Here's how the part is built. I have some questions about the finished solid (model axes, mm). A direction names the side the tool comes from. Round coordinates to 2 decimals unless told otherwise and drop trailing zeros. Loops run counter-clockwise (first coordinate to the right, second up) from the corner with the lowest first, then second, coordinate; pieces in that order, holes last. Notation, with made-up numbers: M 23,34.5 L 35,34.5 A15 cw 35,49.5 Z; hole C 27,-14 d10. An arc over 180 degrees is marked long. Use a Markdown table: item, result.
```python
from build123d import *

# Parameters (mm, degrees)
SKETCH1_W                                      = 45
SKETCH1_H                                      = 35
BOSS_EXTRUDE1_DEPTH                            = 3
CSK_FOR_M3_FLAT_HEAD_MACHINE_SCREW2_AT_2_COUNT = 2
CSK_FOR_M3_FLAT_HEAD_MACHINE_SCREW2_AT_2_PITCH = 20
CSK_FOR_M3_FLAT_HEAD_MACHINE_SCREW2_AT_3_COUNT = 2
CSK_FOR_M3_FLAT_HEAD_MACHINE_SCREW2_AT_3_PITCH = 28.284271247
CSK_FOR_M3_FLAT_HEAD_MACHINE_SCREW2_AT_4_COUNT = 2
CSK_FOR_M3_FLAT_HEAD_MACHINE_SCREW2_AT_4_PITCH = 20
SKETCH7_W                                      = 10
SKETCH7_H                                      = 4
BOSS_EXTRUDE2_DEPTH                            = 50
FILLET1_R                                      = 2
SKETCH12_W                                     = 10
SKETCH12_H                                     = 10
BOSS_EXTRUDE3_DEPTH                            = 15


with BuildPart() as part:
    # Sketch1 → Boss-Extrude1 (new body)
    with BuildSketch(Plane(origin=(0, 0, 0), x_dir=(1, 0, 0), z_dir=(0, 1, 0))):
        Rectangle(SKETCH1_W, SKETCH1_H)
    extrude(amount=BOSS_EXTRUDE1_DEPTH)

    # Sketch5 → CSK for M3 Flat Head Machine Screw2 (revolve, cut)
    with BuildSketch(Plane(origin=(10, 3, -10), x_dir=(0, 0, 1), z_dir=(1, 0, 0))):
        Polygon((0, 0), (0, 3), (1.7, 3), (1.7, 1.45), (3.15, 0), align=None)
    csk_for_m3_flat_head_machine_screw2 = revolve(axis=Axis((10, 9.35, -10), (0, -1, 0)), mode=Mode.SUBTRACT)

    # CSK for M3 Flat Head Machine Screw2 at 2: CSK for M3 Flat Head Machine Screw2 ×2
    with Locations(*[(-i * CSK_FOR_M3_FLAT_HEAD_MACHINE_SCREW2_AT_2_PITCH, 0, 0) for i in range(1, CSK_FOR_M3_FLAT_HEAD_MACHINE_SCREW2_AT_2_COUNT)]):
        add(csk_for_m3_flat_head_machine_screw2, mode=Mode.SUBTRACT)

    # CSK for M3 Flat Head Machine Screw2 at 3: CSK for M3 Flat Head Machine Screw2 ×2
    with Locations(*[Vector(-0.707106781, 0, 0.707106781) * (i * CSK_FOR_M3_FLAT_HEAD_MACHINE_SCREW2_AT_3_PITCH) for i in range(1, CSK_FOR_M3_FLAT_HEAD_MACHINE_SCREW2_AT_3_COUNT)]):
        add(csk_for_m3_flat_head_machine_screw2, mode=Mode.SUBTRACT)

    # CSK for M3 Flat Head Machine Screw2 at 4: CSK for M3 Flat Head Machine Screw2 ×2
    with Locations(*[(0, 0, i * CSK_FOR_M3_FLAT_HEAD_MACHINE_SCREW2_AT_4_PITCH) for i in range(1, CSK_FOR_M3_FLAT_HEAD_MACHINE_SCREW2_AT_4_COUNT)]):
        add(csk_for_m3_flat_head_machine_screw2, mode=Mode.SUBTRACT)

    # Sketch7 → Boss-Extrude2 (add, along a direction that is not the sketch's normal)
    with BuildSketch(Plane(origin=(0, 3, 0), x_dir=(1, 0, 0), z_dir=(0, 1, 0))):
        Rectangle(SKETCH7_W, SKETCH7_H)
    extrude(amount=BOSS_EXTRUDE2_DEPTH, dir=(0, 0.866025404, -0.5))

    # Fillet1
    fillet1_edges = [part.edges().sort_by_distance(p)[0] for p in [
        (22.5, 3, 0),
        (0, 3, -17.5),
        (-22.5, 3, 0),
        (0, 3, 17.5),
        (-22.5, 1.5, -17.5),
        (22.5, 1.5, -17.5),
        (22.5, 1.5, 17.5),
        (-22.5, 1.5, 17.5),
    ]]
    fillet(fillet1_edges, radius=FILLET1_R)

    # Sketch12 → Boss-Extrude3 (add)
    with BuildSketch(Plane(origin=(0, 3, 0), x_dir=(1, 0, 0), z_dir=(0, 1, 0))):
        with Locations((0, 3)):
            Rectangle(SKETCH12_W, SKETCH12_H)
    extrude(amount=BOSS_EXTRUDE3_DEPTH)


solid = part.part
```
Q1. We'd pull the mould along Z, two halves only. Please class faces 1 (the cylindrical face through (21.9, 0.51, -16.93)), 2 (the cylindrical face through (11.5, 0.8, -9.2)), 3 (the cylindrical face through (21.9, 2.43, -0.22)): pulls with the +Z half, pulls with the -Z half, needs draft (parallel to the pull), parting line crosses it, or undercut.
Return value:
| item | result |
|---|---|
| face 1 | pulls with the -Z half |
| face 2 | undercut |
| face 3 | needs draft |
Q2. Imagine slicing it at D-D, the plane x = -1. Please give me the cut outline in (y, z).
Return value:
| item | result |
|---|---|
| outline | M 0,-17.5 L 1,-17.5 A2 ccw 3,-15.5 L 3,-8 L 13.39,-8 L 46.3,-27 L 46.3,-23 L 18,-6.66 L 18,2 L 3,2 L 3,15.5 A2 ccw 1,17.5 L 0,17.5 Z |
Q3. For faces 4 (the cylindrical face through (21.9, 0.51, 16.93)), 5 (the flat face through (0, 10, 2)), 6 (the flat face through (-5, 21, -9)), 7 (the cylindrical face through (0.29, 2.4, -16.93)), which set-ups out of +Z, -Z, +X, -X, +Y, -Y let a thin tool reach every point of the face, with its end or its side?
Return value:
| item | result |
|---|---|
| face 4 | +Z, +X, +Y, -Y |
| face 5 | +Z, +X, -X, +Y |
| face 6 | +Z, -Z, -X, +Y |
| face 7 | -Z, +X, -X |
Q4. Imagine slicing it at A-A, the plane z = 10. Please give me the cut outline in (x, y).
Return value:
| item | result |
|---|---|
| outline | M -22.5,0 L -11.7,0 L -11.7,1.55 L -13.15,3 L -20.5,3 A2 ccw -22.5,1 Z; M -8.3,0 L 8.3,0 L 8.3,1.55 L 6.85,3 L -6.85,3 L -8.3,1.55 Z; M 11.7,0 L 22.5,0 L 22.5,1 A2 ccw 20.5,3 L 13.15,3 L 11.7,1.55 Z |
Q5. Imagine slicing it at B-B, the plane x = 10. Please give me the cut outline in (y, z), then the cut area to 3 significant figures.
Return value:
| item | result |
|---|---|
| outline | M 0,-17.5 L 1,-17.5 A2 ccw 3,-15.5 L 3,-13.15 L 1.55,-11.7 L 0,-11.7 Z; M 0,-8.3 L 1.55,-8.3 L 3,-6.85 L 3,6.85 L 1.55,8.3 L 0,8.3 Z; M 0,11.7 L 1.55,11.7 L 3,13.15 L 3,15.5 A2 ccw 1,17.5 L 0,17.5 Z |
| area | 78.7 mm^2 |
Q6. Imagine slicing it at C-C, the plane z = -10. Please give me the cut outline in (x, y).
Return value:
| item | result |
|---|---|
| outline | M -22.5,0 L -11.7,0 L -11.7,1.55 L -13.15,3 L -20.5,3 A2 ccw -22.5,1 Z; M -8.3,0 L 8.3,0 L 8.3,1.55 L 6.85,3 L -6.85,3 L -8.3,1.55 Z; M -5,16.86 L 5,16.86 L 5,23.78 L -5,23.78 Z; M 11.7,0 L 22.5,0 L 22.5,1 A2 ccw 20.5,3 L 13.15,3 L 11.7,1.55 Z |
Q7. Will these pins go through, and if not, where does the flat tip stop? P1, Ø2.5, axis at x = -10, z = -10, coming from the -Y side; P2, Ø14.5, axis at y = 23.5, z = -18, coming from the +X side; P3, Ø0.8, axis at x = 3.5, y = 0.5, coming from the -Z side; P4, Ø11, axis at x = -1, y = 8, coming from the +Z side.
Return value:
| item | result |
|---|---|
| P1 | passes through |
| P2 | stops at x = 5 |
| P3 | stops at z = -17.5 |
| P4 | stops at z = 16.82 |
Q8. I need wall thicknesses on line 1 (Z direction, x = 10, y = 1.1); line 2 (X direction, y = 1.05, z = -10); line 3 (Y direction, x = -17, z = 8). Which ranges of each line are inside material? Lowest first, please. Write a range as from..to.
Return value:
| item | result |
|---|---|
| line 1 | z = -17.5..-11.7, -8.3..8.3, 11.7..17.5 |
| line 2 | x = -22.5..-11.7, -8.3..8.3, 11.7..22.5 |
| line 3 | y = 0..3 |
